```python
from build123d import *

# Parameters (mm, degrees)
CUT_EXTRUDE1_REACH = 35.675
SKETCH2_R          = 2.5
CUT_EXTRUDE2_DEPTH = 10
SKETCH4_R          = 2.05
CUT_EXTRUDE3_DEPTH = 10


with BuildPart() as part:
    # Sketch1 → Revolve1 (revolve)
    with BuildSketch(Plane(origin=(0, 0, 0), x_dir=(1, 0, 0), z_dir=(0, 1, 0))):
        with BuildLine():
            Line((0, 0), (0, 1))
            Line((0, 1), (7, 1))
            ThreePointArc((7, 1), (7.585786, 2.414214), (9, 3))
            Line((9, 3), (15, 3))
            Line((15, 3), (15, 2))
            Line((15, 2), (9.353553, 2))
            ThreePointArc((9.353553, 2), (8.396447, 1.603553), (8, 0.646447))
            Line((8, 0.646447), (8, 0))
            Line((8, 0), (0, 0))
        make_face()
    revolve(axis=Axis((15, 0, -3), (0, 0, 1)))

    # Cut-Extrude1: up to this face of the body (flat: up to its plane)
    cut_extrude1_end = Plane(part.part.faces().sort_by_distance((29.575736, 0, -1))[0])
    # Sketch2 → Cut-Extrude1 (cut, up to the picked face)
    with BuildSketch(Plane(origin=(0, 0, -3), x_dir=(-1, 0, 0), z_dir=(0, 0, -1)), mode=Mode.PRIVATE) as cut_extrude1_sk1:
        with Locations((-15, 8)):
            Circle(SKETCH2_R)
    cut_extrude1_tool1 = split(extrude(cut_extrude1_sk1.sketch, amount=-CUT_EXTRUDE1_REACH, mode=Mode.PRIVATE), bisect_by=cut_extrude1_end, keep=Keep.BOTH, mode=Mode.PRIVATE)
    # Sketch2 → Cut-Extrude1 (cut, up to the picked face)
    with BuildSketch(Plane(origin=(0, 0, -3), x_dir=(-1, 0, 0), z_dir=(0, 0, -1)), mode=Mode.PRIVATE) as cut_extrude1_sk2:
        with Locations((-7, 0)):
            Circle(SKETCH2_R)
    cut_extrude1_tool2 = split(extrude(cut_extrude1_sk2.sketch, amount=-CUT_EXTRUDE1_REACH, mode=Mode.PRIVATE), bisect_by=cut_extrude1_end, keep=Keep.BOTH, mode=Mode.PRIVATE)
    # Sketch2 → Cut-Extrude1 (cut, up to the picked face)
    with BuildSketch(Plane(origin=(0, 0, -3), x_dir=(-1, 0, 0), z_dir=(0, 0, -1)), mode=Mode.PRIVATE) as cut_extrude1_sk3:
        with Locations((-15, -8)):
            Circle(SKETCH2_R)
    cut_extrude1_tool3 = split(extrude(cut_extrude1_sk3.sketch, amount=-CUT_EXTRUDE1_REACH, mode=Mode.PRIVATE), bisect_by=cut_extrude1_end, keep=Keep.BOTH, mode=Mode.PRIVATE)
    # Sketch2 → Cut-Extrude1 (cut, up to the picked face)
    with BuildSketch(Plane(origin=(0, 0, -3), x_dir=(-1, 0, 0), z_dir=(0, 0, -1)), mode=Mode.PRIVATE) as cut_extrude1_sk4:
        with Locations((-23, 0)):
            Circle(SKETCH2_R)
    cut_extrude1_tool4 = split(extrude(cut_extrude1_sk4.sketch, amount=-CUT_EXTRUDE1_REACH, mode=Mode.PRIVATE), bisect_by=cut_extrude1_end, keep=Keep.BOTH, mode=Mode.PRIVATE)
    add(cut_extrude1_tool1.solids().sort_by(Axis((15, 8, -3), (0, 0, 1)))[0], mode=Mode.SUBTRACT)
    add(cut_extrude1_tool2.solids().sort_by(Axis((7, 0, -3), (0, 0, 1)))[0], mode=Mode.SUBTRACT)
    add(cut_extrude1_tool3.solids().sort_by(Axis((15, -8, -3), (0, 0, 1)))[0], mode=Mode.SUBTRACT)
    add(cut_extrude1_tool4.solids().sort_by(Axis((23, 0, -3), (0, 0, 1)))[0], mode=Mode.SUBTRACT)

    # Sketch3 → Cut-Extrude2 (cut)
    with BuildSketch(Plane(origin=(0, 0, -1), x_dir=(-1, 0, 0), z_dir=(0, 0, -1))):
        with BuildLine():
            ThreePointArc((-12.5, -8), (-15, -5.5), (-17.5, -8))
            ThreePointArc((-17.5, -8), (-17.125, -8.375), (-16.75, -8))
            ThreePointArc((-16.75, -8), (-15, -6.25), (-13.25, -8))
            ThreePointArc((-13.25, -8), (-12.875, -8.375), (-12.5, -8))
        make_face()
        with BuildLine():
            ThreePointArc((-23, -1.75), (-21.25, 0), (-23, 1.75))
            ThreePointArc((-23, 1.75), (-23.375, 2.125), (-23, 2.5))
            ThreePointArc((-23, 2.5), (-20.5, 0), (-23, -2.5))
            ThreePointArc((-23, -2.5), (-23.375, -2.125), (-23, -1.75))
        make_face()
        with BuildLine():
            ThreePointArc((-16.75, 8), (-15, 6.25), (-13.25, 8))
            ThreePointArc((-13.25, 8), (-12.875, 8.375), (-12.5, 8))
            ThreePointArc((-12.5, 8), (-15, 5.5), (-17.5, 8))
            ThreePointArc((-17.5, 8), (-17.125, 8.375), (-16.75, 8))
        make_face()
        with BuildLine():
            ThreePointArc((-7, 1.75), (-8.75, 0), (-7, -1.75))
            ThreePointArc((-7, -1.75), (-6.625, -2.125), (-7, -2.5))
            ThreePointArc((-7, -2.5), (-9.5, 0), (-7, 2.5))
            ThreePointArc((-7, 2.5), (-6.625, 2.125), (-7, 1.75))
        make_face()
    extrude(amount=-CUT_EXTRUDE2_DEPTH, mode=Mode.SUBTRACT)

    # Sketch4 → Cut-Extrude3 (cut)
    with BuildSketch(Plane(origin=(0, 0, -3), x_dir=(-1, 0, 0), z_dir=(0, 0, -1))):
        with Locations((-15, 0)):
            Circle(SKETCH4_R)
    extrude(amount=-CUT_EXTRUDE3_DEPTH, mode=Mode.SUBTRACT)


solid = part.part
```
CAD build for the part. Positions are in the model's coordinates, mm. A direction names the side the tool comes from. Round coordinates to 2 decimals unless told otherwise and drop trailing zeros. Loops run counter-clockwise (first coordinate to the right, second up) from the corner with the lowest first, then second, coordinate; pieces in that order, holes last. Notation, with made-up numbers: (8, 80) - (33, 80) arc R37 ccw to (33, 117) - close; hole circle Ø9 at (84.5, 26.25). An arc over 180 degrees is marked (long way). Return JSON: item names as keys, results as strings. Group by question number.
Q1. Two-plate mould, pull along X, no slides. Class faces 5 (the face through (26.9, 9.13, -0.51)), 6 (the face through (10, -4.9, -0.3)), 7 (the face through (18.1, 6.5, 0)): +X half, -X half, draft (parallel to the pull), parting line (faces both ways), or undercut.
Q2. Band-saw the part on B-B on z = -1.55. Give the cut face in (x, y), plus the area to 3 significant figures.
Q3. Drill centre lines: line 1 along Y through (x, z) = (15, -2.5); line 2 along Z through (x, y) = (26, -8); line 3 along X through (y, z) = (7.25, -1.2). Where is each one in solid material? Low to high. Write a range as [from, to].
Q4. Band-saw the part on C-C on y = -12.25. Give the cut face in (x, z).
Q5. Tool access for faces 1 (the face through (7.635, -1.631, -0.507)), 2 (the face through (19.9, -5, -0.3)), 3 (the face through (12, 0, -3)), 4 (the face through (9, 6, -1)): list every direction of +Z, -Z, +X, -X, +Y, -Y with a clear straight run to the whole face (end or side of a thin tool).
Q6. Band-saw the part on A-A on x = 15. Give the cut face in (y, z).
Q7. Flat gauge pins, fed straight in: pin 1 Ø1.5 at (x, z) = (10, -2) entering from -Y; pin 2 Ø1 at (x, z) = (3, -0.5) entering from +Y; pin 3 Ø3.5 at (x, y) = (15, 0) entering from -Z; pin 4 Ø1.5 at (x, z) = (12, -1) entering from -Y. Where does each tip first touch, or does it go through?
Solutions:
{
 "1": {"face 5": "parting line", "face 6": "undercut", "face 7": "draft"},
 "2": {"outline": "(7.47, -2.46) arc R7.92 ccw to (12.54, -7.53) arc R2.5 cw to (13.1, -6.38) arc R6.65 cw to (8.62, -1.9) arc R2.5 cw to start; (7.47, 2.46) arc R2.5 cw to (8.62, 1.9) arc R6.65 cw to (13.1, 6.38) arc R2.5 cw to (12.54, 7.53) arc R7.92 ccw to start; (16.9, -6.38) arc R2.5 cw to (17.46, -7.53) arc R7.92 ccw to (22.53, -2.46) arc R2.5 cw to (21.38, -1.9) arc R6.65 cw to start; (16.9, 6.38) arc R6.65 cw to (21.38, 1.9) arc R2.5 cw to (22.53, 2.46) arc R7.92 ccw to (17.46, 7.53) arc R2.5 cw to start", "area": "35.1 mm^2"},
 "3": {"line 1": "y = [-5.5, -2.05], [2.05, 5.5]", "line 2": "z = [-1, 0]", "line 3": "x = [11.64, 12.62], [17.38, 18.36]"},
 "4": {"outline": "(6.34, -1) - (23.66, -1) - (23.66, 0) - (6.34, 0) - close"},
 "5": {"face 1": "+Z, -Z", "face 2": "+Z", "face 3": "-Z, +X, -X, +Y, -Y", "face 4": "-Z"},
 "6": {"outline": "(-15, -1) - (-6.95, -1) arc R1.35 cw to (-7, -0.65) - (-7, 0) - (-15, 0) - close; (-5.5, -3) - (-2.05, -3) - (-2.05, -2) - (-5.5, -2) - close; (2.05, -3) - (5.5, -3) - (5.5, -2) - (2.05, -2) - close; (6.95, -1) - (15, -1) - (15, 0) - (7, 0) - (7, -0.65) arc R1.35 cw to start"},
 "7": {"pin 1": "stops at y = -6.59", "pin 2": "stops at y = 9.63", "pin 3": "passes through", "pin 4": "stops at y = -14.83"}
}
